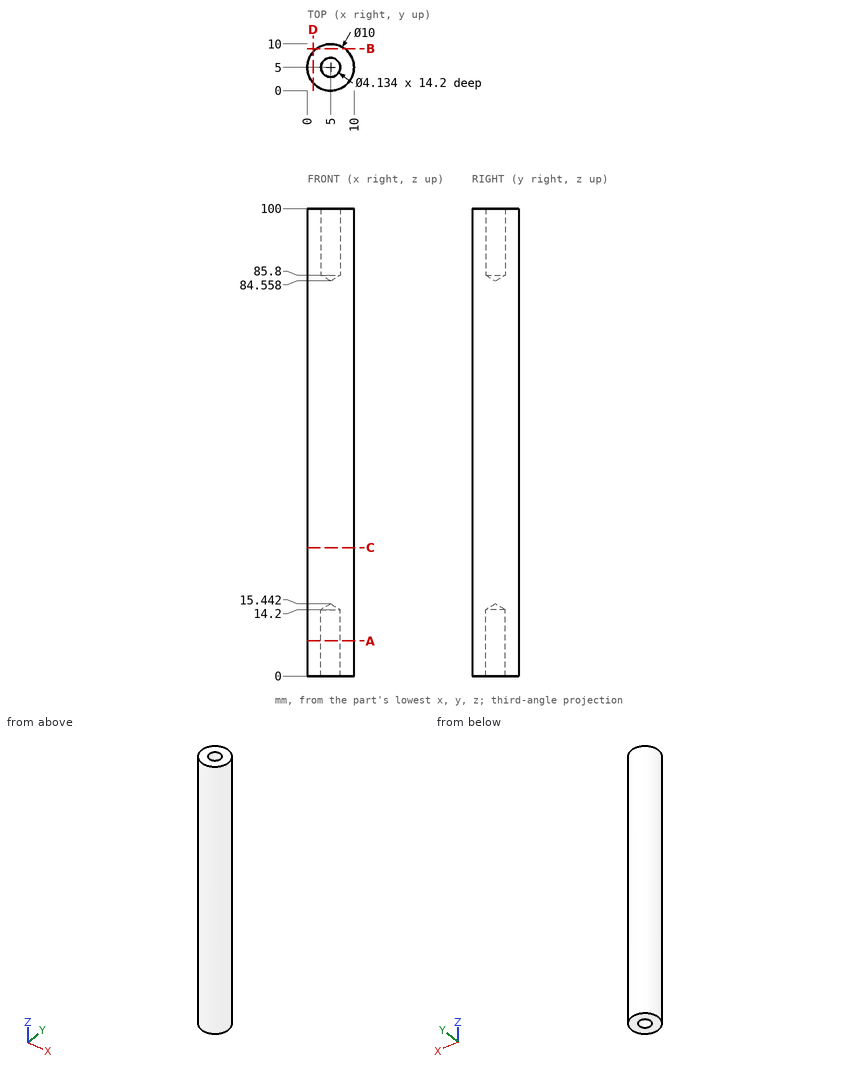
The drawing under review shows one solid part. Ordinate dimensions are in mm from its lowest x, y, z. Coordinates: 2 decimals unless noted, no trailing zeros. Order: outer loops, then holes, each group sorted by start corner. A loop starts at its lowest first (then second) coordinate and runs counter-clockwise, first axis right, second up. Notation, with made-up numbers: (-20, 31.25) -> (22, 31.25) arc R15 cw to (22, 57.25) -> close; hole circle Ø6 at (-20, 52.5). An arc over 180 degrees is marked (long way). Answer in a Markdown table with one row per item.
(1) Consider section C-C (z = 27.5). Write out the cut boundary in (x, y), plus the area to 3 significant figures.
Answers:
| item | result |
|---|---|
| outline | circle Ø10 at (5, 5) |
| area | 78.5 mm² |
(2) Insertion check: pin 1 (3 mm diameter, centred on x = 8.5, z = 23.5, fed in from -Y); pin 2 (5 mm diameter, centred on x = 8.5, y = 3, fed in from -Z); pin 3 (1 mm diameter, centred on y = 7, z = 27, fed in from -X); pin 4 (2.5 mm diameter, centred on x = 5, y = 5, fed in from -Z). Each pin has a flat end and moves straight along its axis. Give the tip position at first contact, or say it passes through.
Answers:
| item | result |
|---|---|
| pin 1 | y = 0.42 |
| pin 2 | z = 0 |
| pin 3 | x = 0.23 |
| pin 4 | z = 14.69 |
(3) Consider section B-B (y = 9). Write out the cut boundary in (x, z), plus the area to 3 significant figures.
Answers:
| item | result |
|---|---|
| outline | (2, 0) -> (8, 0) -> (8, 100) -> (2, 100) -> close |
| area | 600 mm² |
(4) Consider section D-D (x = 1.25). Write out the cut boundary in (y, z).
Answers:
| item | result |
|---|---|
| outline | (1.69, 0) -> (8.31, 0) -> (8.31, 100) -> (1.69, 100) -> close |
(5) Consider section A-A (z = 7.5). Write out the cut boundary in (x, y).
Answers:
| item | result |
|---|---|
| outline | circle Ø10 at (5, 5); hole circle Ø4.13 at (5, 5) |
(6) Wall thickness on line 1 along X through (y, z) = (5, 95); line 2 along X through (y, z) = (8, 17): over which ranges is each line inside the solid? List them lowest first.
Answers:
| item | result |
|---|---|
| line 1 | 0 to 2.93, 7.07 to 10 |
| line 2 | 1 to 9 |
